Design review of the part built by this model. Coordinates are the model's own, in mm. A direction names the side the tool comes from. Round coordinates to 2 decimals unless told otherwise and drop trailing zeros. Loops run counter-clockwise (first coordinate to the right, second up) from the corner with the lowest first, then second, coordinate; pieces in that order, holes last. Notation, with made-up numbers: M -22,29 L 36,29 A16 cw 36,39 Z; hole C 87.25,36.25 d4. An arc over 180 degrees is marked long. Answer as CSV lines item,"result". Start each with the question number.
from build123d import *

# Parameters (mm, degrees)
SKETCH1_R                = 4.5
YOKE_DEPTH               = 23
SKETCH2_R                = 6.75
U_JOINT_BASE_DEPTH       = 3
U_JOINT_STANDUPS_DEPTH   = 9.5
STANDUP_ROUND_DEPTH      = 7.75
STANDUP_ROUND_DEPTH_BACK = 7.75
SKETCH5_R                = 1
BALL_HOLES_DEPTH         = 7.75
BALL_HOLES_DEPTH_BACK    = 7.75
KEYWAY_DEPTH             = 46


with BuildPart() as part:
    # Sketch1 → Yoke (new body, symmetric)
    with BuildSketch(Plane.XY):
        Circle(SKETCH1_R)
    extrude(amount=YOKE_DEPTH, both=True)

    # Sketch2 → U Joint Base (add)
    with BuildSketch(Plane(origin=(0, 0, -23), x_dir=(-1, 0, 0), z_dir=(0, 0, -1))):
        Circle(SKETCH2_R)
    extrude(amount=U_JOINT_BASE_DEPTH)

    # Sketch3 → U Joint Standups (add)
    with BuildSketch(Plane(origin=(0, 0, -26), x_dir=(-1, 0, 0), z_dir=(0, 0, -1))):
        with BuildLine():
            Line((-5.771698, 3.5), (-3.75, 3.5))
            Line((-3.75, 3.5), (-3.75, -3.5))
            Line((-3.75, -3.5), (-5.771698, -3.5))
            ThreePointArc((-5.771698, -3.5), (-6.75, 0), (-5.771698, 3.5))
        make_face()
        with BuildLine():
            Line((3.75, -3.5), (3.75, 3.5))
            Line((3.75, 3.5), (5.771698, 3.5))
            ThreePointArc((5.771698, 3.5), (6.75, 0), (5.771698, -3.5))
            Line((5.771698, -3.5), (3.75, -3.5))
        make_face()
    extrude(amount=U_JOINT_STANDUPS_DEPTH)

    # Sketch4 → Standup Round (cut, two sides)
    with BuildSketch(Plane(origin=(0, 0, 0), x_dir=(0, 0, -1), z_dir=(1, 0, 0))) as standup_round_sk:
        with BuildLine():
            ThreePointArc((32, -3.5), (34.474874, -2.474874), (35.5, 0))
            Line((35.5, 0), (35.5, -3.5))
            Line((35.5, -3.5), (32, -3.5))
        make_face()
        with BuildLine():
            ThreePointArc((35.5, 0), (34.474874, 2.474874), (32, 3.5))
            Line((32, 3.5), (35.5, 3.5))
            Line((35.5, 3.5), (35.5, 0))
        make_face()
    extrude(amount=STANDUP_ROUND_DEPTH, mode=Mode.SUBTRACT)
    extrude(standup_round_sk.sketch, amount=-STANDUP_ROUND_DEPTH_BACK, mode=Mode.SUBTRACT)

    # Sketch5 → Ball Holes (cut, two sides)
    with BuildSketch(Plane(origin=(0, 0, 0), x_dir=(0, 0, -1), z_dir=(1, 0, 0))) as ball_holes_sk:
        with Locations((32, 0)):
            Circle(SKETCH5_R)
    extrude(amount=BALL_HOLES_DEPTH, mode=Mode.SUBTRACT)
    extrude(ball_holes_sk.sketch, amount=-BALL_HOLES_DEPTH_BACK, mode=Mode.SUBTRACT)

    # Sketch6 → Keyway (cut)
    with BuildSketch(Plane.XY.offset(23)):
        Polygon((0.5, -4.472136), (0.5, -4.702036), (-0.5, -4.702036), (-0.5, -4.472136), (-0.5, -3.972136), (0.5, -3.972136), align=None)
    extrude(amount=-KEYWAY_DEPTH, mode=Mode.SUBTRACT)


solid = part.part
Item 1: To check wall thickness, follow line 1 (Z direction, x = -5.65, y = 0); line 2 (Y direction, x = 5.1, z = -32); line 3 (Z direction, x = -1.5, y = -1.75). State the ranges of each line that lie inside material, in increasing order.
Item 2: Insertion check: pin 1 Ø4 at (y, z) = (-2.5, -27.5) entering from +X; pin 2 Ø8 at (y, z) = (-5, -8.5) entering from +X; pin 3 Ø0.6 at (x, z) = (-4.5, -28) entering from +Y. Each pin has a flat end and moves straight along its axis. Give the tip position at first contact, or say it passes through.
Item 3: Tool access review of faces 4 (the face through (-5, 0, -31)), 5 (the face through (3.75, 0, -30.7)), 6 (the face through (-5, 3.5, -29)), 7 (the face through (-5, -3.5, -29)): name each direction out of +Z, -Z, +X, -X, +Y, -Y from which nothing blocks a thin tool from reaching the whole face with its end or side.
Item 4: Consider section B-B, the plane y = -0.5. Write out the cut boundary in (x, z), then the cut area to 3 significant figures.
Item 5: Consider section D-D, the plane z = 8.5. Write out the cut boundary in (x, y).
Item 6: Consider section C-C, the plane x = 0. Write out the cut boundary in (y, z), then the cut area to 3 significant figures.
Item 7: The part is to be moulded in two halves that separate along X. For faces 1 (the face through (5, -3.5, -29)), 2 (the face through (0.191, 4.496, 0.322)), 3 (the face through (0, -3.972, 0)), say which applies: +X half, -X half, draft (parallel to the pull), parting line (faces both ways), or undercut.
Item 8: Consider section A-A, the plane z = -27. Write out the cut boundary in (x, y), then the cut area to 3 significant figures.
Found:
1,line 1,"z = -35.5 to -33, -31 to -23"
1,line 2,"y = -3.5 to -1, 1 to 3.5"
1,line 3,"z = -26 to 23"
2,pin 1,"stops at x = 6.73"
2,pin 2,"stops at x = 4.39"
2,pin 3,"stops at y = 3.5"
3,face 4,"+X, -X"
3,face 5,"-Z, +Y, -Y"
3,face 6,"-Z, +X, -X, +Y"
3,face 7,"-Z, +X, -X, -Y"
4,outline,"M -6.73,-35.46 L -3.75,-35.46 L -3.75,-32.87 L -6.73,-32.87 Z; M -6.73,-31.13 L -3.75,-31.13 L -3.75,-26 L 3.75,-26 L 3.75,-31.13 L 6.73,-31.13 L 6.73,-23 L 4.47,-23 L 4.47,23 L -4.47,23 L -4.47,-23 L -6.73,-23 Z; M 3.75,-35.46 L 6.73,-35.46 L 6.73,-32.87 L 3.75,-32.87 Z"
4,area,"498 mm^2"
5,outline,"M -0.5,-4.47 L -0.5,-3.97 L 0.5,-3.97 L 0.5,-4.47 A4.5 ccw long Z"
6,outline,"M -6.75,-26 L 6.75,-26 L 6.75,-23 L 4.5,-23 L 4.5,23 L -3.97,23 L -3.97,-23 L -6.75,-23 Z"
6,area,"430 mm^2"
7,face 1,"draft"
7,face 2,"parting line"
7,face 3,"undercut"
8,outline,"M -5.77,-3.5 L -3.75,-3.5 L -3.75,3.5 L -5.77,3.5 A6.75 ccw Z; M 3.75,-3.5 L 5.77,-3.5 A6.75 ccw 5.77,3.5 L 3.75,3.5 Z"
8,area,"37.6 mm^2"
